Can you work these out from the model? Positions are in its coordinate system, mm. Face numbers are marked on the shaded views. A direction names the side the tool comes from. Give positions to 0.01 mm unless a question says otherwise; leave off trailing zeros. Order: outer loops, then holes, each group sorted by start corner. A loop starts at its lowest first (then second) coordinate and runs counter-clockwise, first axis right, second up.
Item 1: I want a section at B-B, the plane x = 7.75. Write out the boundary of the cut face in (y, z).
Item 2: I'm going to push a flat-ended pin straight in: pin 1 Ø1.5 at (x, y) = (1.5, 5.5) entering from +Z. Where does the tip first touch, or does it pass through?
Item 3: I want a section at C-C, the plane y = 4. Write out the boundary of the cut face in (x, z).
Item 4: Which directions (+Z, -Z, +X, -X, +Y, -Y) give clear straight access to the entire face, cutting with the end or side of a thin tool? Please do the marked faces 1 and 2.
Item 5: If I drill on line 1 along Y through (x, z) = (6.25, 0); line 2 along Z through (x, y) = (0, 3.95), over which ranges is the centre line in solid material (lowest first)?
Item 6: I want a section at A-A, the plane z = 0. Write out the boundary of the cut face in (x, y).
```python
from build123d import *

# Parameters (mm, degrees)
SKETCH1_R           = 0.45
SKETCH1_R_2         = 0.25
REVOLVE1_ANGLE      = 90
SKETCH6_R           = 0.45
BOSS_EXTRUDE1_DEPTH = 6
SKETCH11_R          = 0.45
BOSS_EXTRUDE2_DEPTH = 9
SKETCH17_W          = 9
SKETCH17_H          = 0.25
SKETCH19_W          = 0.25
SKETCH19_H          = 6


with BuildPart() as part:
    # Sketch1 → Revolve1 (revolve)
    with BuildSketch(Plane(origin=(1, 0, 0), x_dir=(0, 0, -1), z_dir=(1, 0, 0))):
        with Locations((0, 7)):
            Circle(SKETCH1_R)
        with Locations((0, 7)):
            Circle(SKETCH1_R_2, mode=Mode.SUBTRACT)
    revolve(axis=Axis((1, 6, 0.4), (0, 0, 1)), revolution_arc=REVOLVE1_ANGLE)

    # Sketch6 → Boss-Extrude1 (add)
    with BuildSketch(Plane(origin=(0, 6, 0), x_dir=(-1, 0, 0), z_dir=(0, -1, 0))):
        Circle(SKETCH6_R)
    extrude(amount=BOSS_EXTRUDE1_DEPTH)

    # Sketch11 → Boss-Extrude2 (add)
    with BuildSketch(Plane(origin=(1, 0, 0), x_dir=(0, 0, -1), z_dir=(1, 0, 0))):
        with Locations((0, 7)):
            Circle(SKETCH11_R)
    extrude(amount=BOSS_EXTRUDE2_DEPTH)

    # Sketch17 → Cut-Revolve1 (revolve, cut)
    with BuildSketch(Plane(origin=(0, 0, 0), x_dir=(-1, 0, 0), z_dir=(0, 0, -1))):
        with Locations((-5.5, 7.125)):
            Rectangle(SKETCH17_W, SKETCH17_H)
    revolve(axis=Axis((10, 7, 0), (-1, 0, 0)), mode=Mode.SUBTRACT)

    # Sketch19 → Cut-Revolve2 (revolve, cut)
    with BuildSketch(Plane.XY):
        with Locations((0.125, 3)):
            Rectangle(SKETCH19_W, SKETCH19_H)
    revolve(axis=Axis((0, 6, 0), (0, -1, 0)), mode=Mode.SUBTRACT)


solid = part.part
```
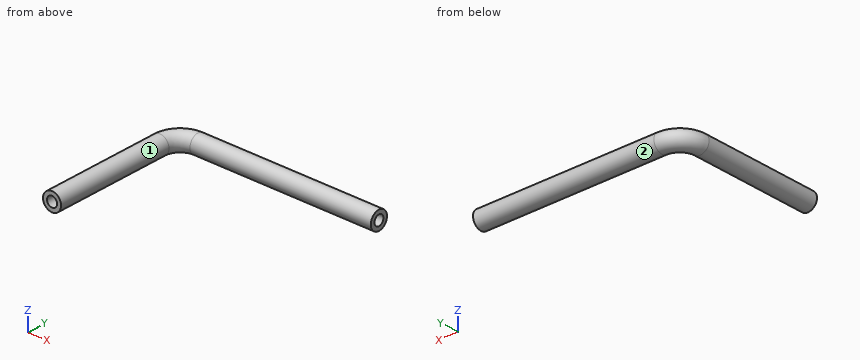
Results list:
1. outline: circle Ø0.9 at (7, 0); hole circle Ø0.5 at (7, 0)
2. pin 1: passes through
3. outline: circle Ø0.9 at (0, 0); hole circle Ø0.5 at (0, 0)
4. face 1: -Y
4. face 2: +X
5. line 1: y = 6.55 to 6.75, 7.25 to 7.45
5. line 2: z = -0.45 to -0.25, 0.25 to 0.45
6. outline: (-0.45, 0) - (-0.25, 0) - (-0.25, 6) arc R1.25 cw to (1, 7.25) - (10, 7.25) - (10, 7.45) - (1, 7.45) arc R1.45 ccw to (-0.45, 6) - close; (0.25, 0) - (0.45, 0) - (0.45, 6) arc R0.55 cw to (1, 6.55) - (10, 6.55) - (10, 6.75) - (1, 6.75) arc R0.75 ccw to (0.25, 6) - close
